Here's how the part is built. I have some questions about the finished solid (model axes, mm). Face numbers are marked on the shaded views. A direction names the side the tool comes from. Coordinates: 2 decimals unless noted, no trailing zeros. Order: outer loops, then holes, each group sorted by start corner. A loop starts at its lowest first (then second) coordinate and runs counter-clockwise, first axis right, second up. Notation, with made-up numbers: (50.5, 5.25) - (68.5, 5.25) arc R24 cw to (68.5, 21.25) - close; hole circle Ø7 at (14.25, 87.5). An arc over 180 degrees is marked (long way). Answer in a Markdown table with one row per item. Add a question column.
Item 1: On a 3-axis mill with a long thin cutter (end or side, diameter ignored), from which of +Z, -Z, +X, -X, +Y, -Y can I reach the whole of each face in a straight line? I mean the marked faces 4, 5, 6, 7 and 8. Say none if no direction works.
Item 2: If I drill on line 1 along Z through (x, y) = (11.5, -9.25); line 2 along Z through (x, y) = (4.25, -10.25); line 3 along Z through (x, y) = (2, -2.5), over which ranges is the centre line in solid material (lowest first)? Write a range as from..to.
Item 3: I want a section at C-C (y = -14.75). Please give me the cut outline in (x, z).
Item 4: I want a section at D-D (y = -3.5). Please give me the cut outline in (x, z).
Item 5: Thinking about a two-plate mould opening in X: for the marked faces 1, 2 and 3, which applies, +X half, -X half, draft (parallel to the pull), parting line (faces both ways), or undercut?
Item 6: I want a section at B-B (z = -35). Please give me the cut outline in (x, y), plus the area to 4 significant figures.
Item 7: Will these pins go through, and if not, where does the flat tip stop? pin 1 Ø1 at (y, z) = (-11.5, -21) entering from +X; pin 2 Ø1 at (x, z) = (6, -32.5) entering from -Y.
Item 8: I want a section at A-A (x = 7). Please give me the cut outline in (y, z), plus the area to 3 significant figures.
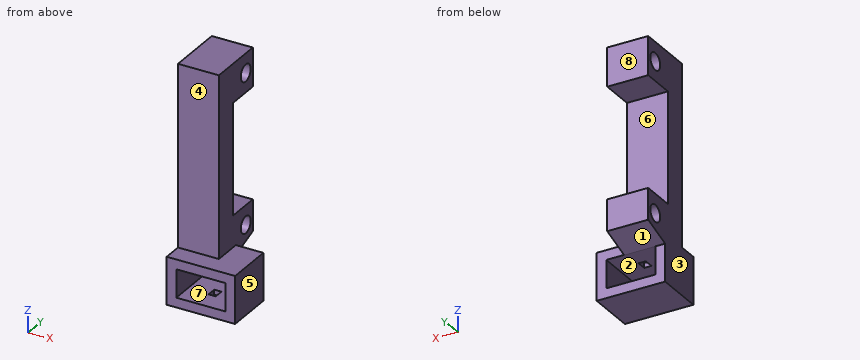
Autodesk Inventor part; units mm, degrees
ref_plane "YZ Plane" through (0, 0, 0) normal (1, 0, 0) x (0, 1, 0)
ref_plane "XZ Plane" through (0, 0, 0) normal (0, 1, 0) x (-1, 0, 0)
ref_plane "XY Plane" through (0, 0, 0) normal (0, 0, 1) x (1, 0, 0)
sketch "Sketch1" plane through (0, 0, 0) normal (1, 0, 0) x (0, 1, 0)
  line L0 (0, 0) -> (0, -8)
  line L1 (0, -8) -> (-7, -8)
  line L2 (-7, -8) -> (-7, -31)
  line L3 (-7, -31) -> (0, -31)
  line L4 (0, -31) -> (0, -37.5)
  line L5 (0, -37.5) -> (-12, -37.5)
  line L6 (-12, -37.5) -> (-12, 0)
  line L7 (-12, 0) -> (0, 0)
  line L8 (0, -4) -> (-2.5, -4) construction
  circle A0 centre (-2.5, -4) radius 1.75
  line L9 (0, -31) -> (-2.5, -31) construction
  line L10 (-2.5, -31) -> (-2.5, -35) construction
  circle A1 centre (-2.5, -35) radius 1.75
  dimension "d0" = 8
  dimension "d1" = 7
  dimension "d2" = 23
  dimension "d3" = 6.5
  dimension "d4" = 12
  dimension "d5" = 2.5
  dimension "d6" = 3.5
  dimension "d7" = 4
  dimension "d8" = 3.5
extrude "Extrusion1" add sketch "Sketch1" along normal blind 8.5
sketch "Sketch2" plane through (0, 0, -31) normal (0, 1, 0) x (1, 0, 0)
  line L0 (0, 6.5) -> (0, -31)
  line L1 (0, 6.5) -> (2, 6.5) construction
  line L2 (0, 6.5) -> (8.5, 6.5) construction
  line L3 (2, 6.5) -> (0, 6.5) construction
  line L4 (0, 16.3) -> (2, 16.3) construction
  line L5 (2, 16.3) -> (2, 14.3) construction
  line L6 (2, 14.3) -> (12.2, 14.3)
  line L7 (12.2, 14.3) -> (12.2, 8.5)
  line L8 (12.2, 8.5) -> (2, 8.5)
  line L9 (2, 8.5) -> (2, 14.3)
  line L10 (0, 6.5) -> (14.2, 6.5)
  line L11 (14.2, 6.5) -> (14.2, 16.3)
  line L12 (14.2, 16.3) -> (0, 16.3)
  line L13 (0, 16.3) -> (0, 6.5)
  dimension "d11" = 9.8
  dimension "d15" = 2
  dimension "d16" = 2
  dimension "d17" = 10.2
  dimension "d18" = 5.8
  dimension "d19" = 14.2
extrude "Extrusion2" add sketch "Sketch2" against normal blind 16
extrude "Extrusion3" cut sketch "Sketch2" against normal blind 6
sketch "Sketch3" plane through (8.5, 0, 0) normal (1, 0, 0) x (0, 0, -1)
  line L0 (37.5, 0) -> (31, 0)
  line L1 (37.5, 0) -> (39.5451, -6)
  line L2 (37.5, -12) -> (37.5, -6)
  line L3 (39.5451, -6) -> (37.5, -6)
  line L4 (37.5, -6) -> (37.5, 0)
  point P0 (0, 0)
extrude "Extrusion4" add sketch "Sketch3" against normal blind 8.5
sketch "Sketch4" plane through (2, -16, -45.3) normal (0, 0, 1) x (1, 0, 0)
  line L0 (10.2, 0) -> (0, 0) construction
  line L1 (5.1, 0) -> (5.1, 4) construction
  line L2 (10.2, 10) -> (0, 10) construction
  line L3 (5.1, 4) -> (4.35, 4) construction
  line L4 (4.35, 4) -> (5.85, 4)
  line L5 (5.85, 4) -> (5.85, 6)
  line L6 (5.85, 6) -> (4.35, 6)
  line L7 (4.35, 6) -> (4.35, 4)
  point P0 (-2, 16)
  dimension "d28" = 1.5
  dimension "d29" = 2
extrude "Extrusion5" cut sketch "Sketch4" against normal blind 1
sketch "Sketch5" plane through (12.2, -16, -39.5) normal (0, 0, -1) x (-1, 0, 0)
  line L0 (10.2, 0) -> (0, 0) construction
  line L1 (5.1, 0) -> (5.1, 4) construction
  line L2 (5.1, 4) -> (4.35, 4) construction
  line L3 (4.35, 4) -> (5.85, 4)
  line L4 (5.85, 4) -> (5.85, 6)
  line L5 (5.85, 6) -> (4.35, 6)
  line L6 (4.35, 6) -> (4.35, 4)
  point P0 (12.2, 16)
  dimension "d34" = 1.5
  dimension "d35" = 2
extrude "Extrusion6" cut sketch "Sketch5" against normal blind 1
properties part number "Proximity Sensor Mount_1"
Values follow:
| question | item | result |
|---|---|---|
| 1 | face 4 | +Z, +X, -X, -Y |
| 1 | face 5 | +Z, -Z, +X, +Y, -Y |
| 1 | face 6 | +X, -X, +Y |
| 1 | face 7 | +Y, -Y |
| 1 | face 8 | +Z, -Z, +X, -X, +Y |
| 2 | line 1 | z = -47.3..-45.3, -39.5..-37.5 |
| 2 | line 2 | z = -47.3..-45.3, -39.5..0 |
| 2 | line 3 | z = -38.35..-36.75, -33.25..-31, -8..-5.75, -2.25..0 |
| 3 | outline | (0, -47.3) - (14.2, -47.3) - (14.2, -37.5) - (0, -37.5) - close; hole (2, -45.3) - (12.2, -45.3) - (12.2, -39.5) - (2, -39.5) - close |
| 4 | outline | (0, -38.69) - (8.5, -38.69) - (8.5, -36.44) - (0, -36.44) - close; (0, -33.56) - (8.5, -33.56) - (8.5, -31) - (0, -31) - close; (0, -8) - (8.5, -8) - (8.5, -5.44) - (0, -5.44) - close; (0, -2.56) - (8.5, -2.56) - (8.5, 0) - (0, 0) - close |
| 5 | face 1 | draft |
| 5 | face 2 | undercut |
| 5 | face 3 | -X half |
| 6 | outline | (0, -12) - (8.5, -12) - (8.5, -4.25) - (0, -4.25) - close; (0, -0.75) - (8.5, -0.75) - (8.5, 0) - (0, 0) - close |
| 6 | area | 72.25 mm^2 |
| 7 | pin 1 | stops at x = 8.5 |
| 7 | pin 2 | stops at y = -12 |
| 8 | outline | (-16, -47.3) - (-6, -47.3) - (-6, -45.3) - (-10, -45.3) - (-10, -46.3) - (-12, -46.3) - (-12, -45.3) - (-16, -45.3) - close; (-16, -39.5) - (-12, -39.5) - (-12, -38.5) - (-10, -38.5) - (-10, -39.5) - (-6, -39.5) - (-6, -39.55) - (0, -37.5) - (0, -31) - (-7, -31) - (-7, -8) - (0, -8) - (0, 0) - (-12, 0) - (-12, -37.5) - (-16, -37.5) - close; hole circle Ø3.5 at (-2.5, -35); hole circle Ø3.5 at (-2.5, -4) |
| 8 | area | 312 mm^2 |
